```python
from build123d import *

# Parameters (mm, degrees)
F0_R        = 20.565163
F0_R_2      = 17.333449
F1_DEPTH    = 250
F2_R        = 19.942448
F3_DEPTH    = 5
F4_R        = 19.942448
F4_R_2      = 3.853128
F3_FACE_R   = 19.942448
F3_FACE_R_2 = 17.333449
F5_DEPTH    = 25
F6_R        = 4.28003
F7_DEPTH    = 153
F8_W        = 454.783313
F8_H        = 260.354363
F9_DEPTH    = 142


with BuildPart() as f1:
    # F0 (on Front) → F1 (new body)
    with BuildSketch(Plane.XZ):
        Circle(F0_R)
        Circle(F0_R_2, mode=Mode.SUBTRACT)
    extrude(amount=F1_DEPTH)

    # F2 (on Front) → F3 (join)
    with BuildSketch(Plane.XZ):
        Circle(F2_R)
    extrude(amount=-F3_DEPTH)

    # F4 (on face) + F3_face (on face) → F5 (join)
    with BuildSketch(Plane(origin=(0, 5, 0), x_dir=(-1, 0, 0), z_dir=(0, 1, 0))):
        Circle(F4_R)
        Circle(F4_R_2, mode=Mode.SUBTRACT)
        Circle(F4_R_2)
    with BuildSketch(Plane(origin=(0, 5, 0), x_dir=(1, 0, 0), z_dir=(0, 1, 0))):
        Circle(F3_FACE_R)
        Circle(F3_FACE_R_2)
    extrude(amount=F5_DEPTH)

    # F6 (on face) → F7 (cut)
    with BuildSketch(Plane(origin=(0, 30, 0), x_dir=(-1, 0, 0), z_dir=(0, 1, 0))):
        Circle(F6_R)
    extrude(amount=-F7_DEPTH, mode=Mode.SUBTRACT)

    # F8 (on Right) → F9 (cut)
    with BuildSketch(Plane.YZ):
        with Locations((-137.636367, 25.624771)):
            Rectangle(F8_W, F8_H)
    extrude(amount=-F9_DEPTH, mode=Mode.SUBTRACT)


solid = f1.part
```
Design review of the part built by this model. Coordinates are the model's own, in mm. A direction names the side the tool comes from. Round coordinates to 2 decimals unless told otherwise and drop trailing zeros. Order: outer loops, then holes, each group sorted by start corner. A loop starts at its lowest first (then second) coordinate and runs counter-clockwise, first axis right, second up. Notation, with made-up numbers: M -36.5,20.5 L 8.5,20.5 A23 cw 8.5,37.5 Z; hole C -4.5,-26 d2. An arc over 180 degrees is marked long. Put each result on its own line as item: value.
Q1. Consider section A-A (z = 0). State the section outline as (x, y) points, and give its area (3 significant figures).
Reported:
outline: M 4.28,0 L 17.33,0 L 17.33,-250 L 20.57,-250 L 20.57,0 L 19.94,0 L 19.94,30 L 4.28,30 Z
area: 1,280 mm²
Q2. Machinability: for faces 4 (the face through (4.28, 15.21, 0.09)), 5 (the face through (20.1, 0, 0.1)), 6 (the face through (17.33, -123.25, -0.38)), which of the approach directions +Z, -Z, +X, -X, +Y, -Y give a long, thin tool a straight path to every point of the face, cutting with its end or side? Answer none if there is none.
Reported:
face 4: -X, +Y, -Y
face 5: +X, +Y
face 6: -X, -Y
Q3. To check wall thickness, follow line 1 (Z direction, x = 1, y = -135); line 2 (Y direction, x = 15.25, z = 13); line 3 (Y direction, x = 6, z = 3). State the ranges of each line that lie inside material, in increasing order.
Reported:
line 1: -20.54 to -17.3, 17.3 to 20.54
line 2: -250 to 0
line 3: 0 to 30
Q4. Draft analysis for pull direction Z (two halves, no side actions). For faces 1 (the face through (20.56, -123.25, -0.45)), 2 (the face through (0, -69, -18)), 3 (the face through (9, 0, 0)), state which applies: released by +Z, released by -Z, zero draft, split by the parting line, or undercut.
Reported:
face 1: split by the parting line
face 2: zero draft
face 3: undercut
Q5. Consider section C-C (y = -139). State the section outline as (x, z) points, and give its area (3 significant figures).
Reported:
outline: M 0,-20.57 A20.57 ccw 0,20.57 L 0,17.33 A17.33 cw 0,-17.33 Z
area: 192 mm²
Q6. Consider section B-B (x = 9.25). State the section outline as (y, z) points, and give its area (3 significant figures).
Reported:
outline: M -250,-18.37 L 0,-18.37 L 0,-17.67 L 30,-17.67 L 30,17.67 L 0,17.67 L 0,18.37 L -250,18.37 L -250,14.66 L 0,14.66 L 0,-14.66 L -250,-14.66 Z
area: 2,910 mm²
Q7. Insertion check: pin 1 Ø1 at (x, y) = (13.5, -43.5) entering from -Z; pin 2 Ø1.5 at (y, z) = (-184, 0) entering from +X; pin 3 Ø8 at (y, z) = (-18.5, -8) entering from +X. Each pin has a flat end and moves straight along its axis. Give the tip position at first contact, or say it passes through.
Reported:
pin 1: z = -15.94
pin 2: x = 20.57
pin 3: x = 20.17
Q8. Consider section D-D (z = -14). State the section outline as (x, y) points, and give its area (3 significant figures).
Reported:
outline: M 0,0 L 10.22,0 L 10.22,-250 L 15.06,-250 L 15.06,0 L 14.2,0 L 14.2,30 L 0,30 Z
area: 1,640 mm²
